```python
from build123d import *

# Parameters (mm, degrees)
F0_W     = 12.7
F0_H     = 12.7
F1_DEPTH = 152.4
F2_W     = 107.95
F2_H     = 139.7
F3_DEPTH = 38.1
F5_DEPTH = 6.35


with BuildPart() as f1:
    # F0 (on Front) → F1 (new body)
    with BuildSketch(Plane.XZ):
        Polygon((56.291819, 19.05), (-64.358181, 19.05), (-64.358181, 0), (-64.358181, -12.7), (-64.358181, -31.75), (56.291819, -31.75), (56.291819, -12.7), (56.291819, 0), align=None)
        with Locations((-70.708181, -6.35)):
            Rectangle(F0_W, F0_H)
        with Locations((62.641819, -6.35)):
            Rectangle(F0_W, F0_H)
    extrude(amount=F1_DEPTH)

    # F2 (on face) → F3 (cut)
    with BuildSketch(Plane.XY.offset(19.05)):
        with Locations((-4.033181, -76.2)):
            Rectangle(F2_W, F2_H)
    extrude(amount=-F3_DEPTH, mode=Mode.SUBTRACT)

    # F4 (on face) → F5 (cut)
    with BuildSketch(Plane.XZ.offset(152.4)):
        with BuildLine():
            Line((0, 19.05), (-15.476204, 19.05))
            ThreePointArc((-15.476204, 19.05), (-7.738102, 13.646425), (0, 19.05))
        make_face()
    extrude(amount=-F5_DEPTH, mode=Mode.SUBTRACT)


solid = f1.part
```
Verification items for the finished model (mm, model axes). A direction names the side the tool comes from. Coordinates: 2 decimals unless noted, no trailing zeros. Order: outer loops, then holes, each group sorted by start corner. A loop starts at its lowest first (then second) coordinate and runs counter-clockwise, first axis right, second up. Notation, with made-up numbers: (11.25, 82) - (45.25, 82) arc R21 cw to (45.25, 118) - close; hole circle Ø3 at (-23, -8.75). An arc over 180 degrees is marked (long way). Return JSON: item names as keys, results as strings.
(1) Access from +Z, -Z, +X, -X, +Y, -Y to the whole of each face (thin tool, end or side, straight path). Record for faces 1 (the cylindrical face through (-7.879, -149.269, 13.648)), 2 (the flat face through (-5, -75, -19.05)), 3 (the flat face through (63, -75, 0)), 4 (the flat face through (-64.358, -75, 10)).
Filled sheet:
{"face 1": "+Z, -Y", "face 2": "+Z", "face 3": "+Z, +X, +Y, -Y", "face 4": "+Z, -X, +Y, -Y"}
(2) Section check D-D, the plane z = -8. Record the cut outline in (x, y).
Filled sheet:
{"outline": "(-77.06, -152.4) - (68.99, -152.4) - (68.99, 0) - (-77.06, 0) - close; hole (-58.01, -146.05) - (49.94, -146.05) - (49.94, -6.35) - (-58.01, -6.35) - close"}
(3) Thickness scan on line 1 along Y through (x, z) = (27, -19); line 2 along X through (y, z) = (-104, -0.5); line 3 along X through (y, z) = (-124, 14.5). Record the ranges inside material, lowest first.
Filled sheet:
{"line 1": "y = -152.4 to -146.05, -6.35 to 0", "line 2": "x = -77.06 to -58.01, 49.94 to 68.99", "line 3": "x = -64.36 to -58.01, 49.94 to 56.29"}
(4) Section check C-C, the plane y = -16.5. Record the cut outline in (x, z), and give its area (3 significant figures).
Filled sheet:
{"outline": "(-77.06, -12.7) - (-64.36, -12.7) - (-64.36, -31.75) - (56.29, -31.75) - (56.29, -12.7) - (68.99, -12.7) - (68.99, 0) - (56.29, 0) - (56.29, 19.05) - (49.94, 19.05) - (49.94, -19.05) - (-58.01, -19.05) - (-58.01, 19.05) - (-64.36, 19.05) - (-64.36, 0) - (-77.06, 0) - close", "area": "2,340 mm^2"}
(5) Section check B-B, the plane x = 10. Record the cut outline in (y, z), and give its area (3 significant figures).
Filled sheet:
{"outline": "(-152.4, -31.75) - (0, -31.75) - (0, 19.05) - (-6.35, 19.05) - (-6.35, -19.05) - (-146.05, -19.05) - (-146.05, 19.05) - (-152.4, 19.05) - close", "area": "2,420 mm^2"}
(6) Go/stop test with flat-tipped pins: pin 1 (10 mm diameter, centred on x = -33, y = -98.5, fed in from +Z); pin 2 (6.5 mm diameter, centred on x = 60, y = -46, fed in from +Z); pin 3 (9.5 mm diameter, centred on y = -42.5, z = 11.5, fed in from +X). Record where each tip stops, or that it passes through.
Filled sheet:
{"pin 1": "stops at z = -19.05", "pin 2": "stops at z = 0", "pin 3": "stops at x = 56.29"}
(7) Mould release check, pull along Y, two halves, no side actions. Record for faces 5 (the flat face through (-5, -6.35, 0)), 6 (the flat face through (56.292, -75, 9)), 7 (the flat face through (-5, -152.4, -6)): pulls with the +Y half, pulls with the -Y half, needs draft (parallel to the pull), parting line crosses it, or undercut.
Filled sheet:
{"face 5": "undercut", "face 6": "needs draft", "face 7": "pulls with the -Y half"}
(8) Section check A-A, the plane z = 9.5. Record the cut outline in (x, y).
Filled sheet:
{"outline": "(-64.36, -152.4) - (56.29, -152.4) - (56.29, 0) - (-64.36, 0) - close; hole (-58.01, -146.05) - (49.94, -146.05) - (49.94, -6.35) - (-58.01, -6.35) - close"}
